The listing builds one solid part. Answer for the finished solid, in the listing's coordinates (mm). Give positions to 0.01 mm unless a question says otherwise; leave off trailing zeros. Loops run counter-clockwise (first coordinate to the right, second up) from the corner with the lowest first, then second, coordinate; pieces in that order, holes last. Notation, with made-up numbers: (9.25, 12) - (41.25, 12) arc R21 ccw to (41.25, 40) - close; hole circle Ø1 at (48, 9.5). An arc over 180 degrees is marked (long way). Write each question's results on one line, items separated by ' | '.
from build123d import *

# Parameters (mm, degrees)
SKETCH1_W           = 24
SKETCH1_H           = 30
BOSS_EXTRUDE1_DEPTH = 1.5
SKETCH2_R           = 1.55
CUT_EXTRUDE1_DEPTH  = 3
FILLET1_R           = 10
FILLET2_R           = 2


with BuildPart() as part:
    # Sketch1 → Boss-Extrude1 (new body, symmetric)
    with BuildSketch(Plane(origin=(0, 0, 0), x_dir=(1, 0, 0), z_dir=(0, 1, 0))):
        Polygon((-92, -95), (-92, -115), (12, -15), (-12, -15), (-12, 15), align=None)
        Rectangle(SKETCH1_W, SKETCH1_H)
    extrude(amount=BOSS_EXTRUDE1_DEPTH, both=True)

    # Sketch2 → Cut-Extrude1 (cut)
    with BuildSketch(Plane(origin=(0, 1.5, 0), x_dir=(1, 0, 0), z_dir=(0, 1, 0))):
        with Locations((6, 0)):
            Circle(SKETCH2_R)
        with Locations((-2, 0)):
            Circle(SKETCH2_R)
        with Locations((-47, -55)):
            Circle(SKETCH2_R)
    extrude(amount=-CUT_EXTRUDE1_DEPTH, mode=Mode.SUBTRACT)

    # Fillet1
    fillet1_edges = [part.edges().sort_by_distance(p)[0] for p in [
        (-92, 0, 95),
    ]]
    fillet(fillet1_edges, radius=FILLET1_R)

    # Fillet2
    fillet2_edges = [part.edges().sort_by_distance(p)[0] for p in [
        (-92, 0, 115),
    ]]
    fillet(fillet2_edges, radius=FILLET2_R)


solid = part.part
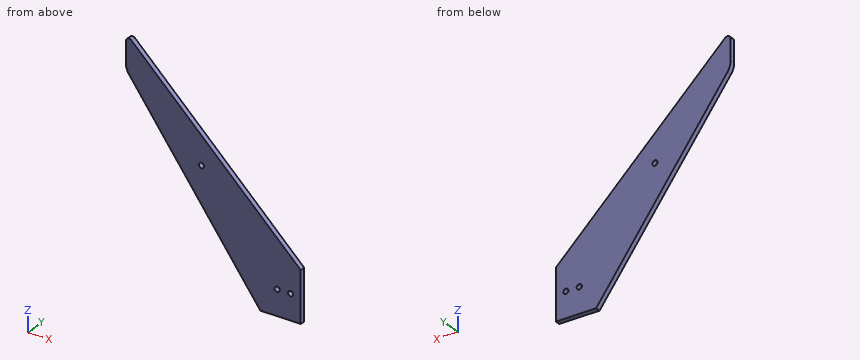
Item 1: A cutting plane is placed at C-C, the plane z = 0. Determine the outline of the cut face in (x, y), plus the area to 3 significant figures.
Values found:
outline: (-22.91, -1.5) - (-3.55, -1.5) - (-3.55, 1.5) - (-22.91, 1.5) - close; (-0.45, -1.5) - (4.45, -1.5) - (4.45, 1.5) - (-0.45, 1.5) - close; (7.55, -1.5) - (12, -1.5) - (12, 1.5) - (7.55, 1.5) - close | area: 86.1 mm²
Item 2: A cutting plane is placed at A-A, the plane y = 0.9. Determine the outline of the cut face in (x, z), plus the area to 3 significant figures.
Values found:
outline: (-92, 98.25) arc R10 ccw to (-90.09, 92.37) - (-12, -15) - (12, -15) - (12, 15) - (-88.61, 111.74) arc R2 ccw to (-92, 110.3) - close; hole circle Ø3.1 at (-47, 55); hole circle Ø3.1 at (-2, 0); hole circle Ø3.1 at (6, 0) | area: 3,890 mm²
Item 3: Find the intervals of material crossed by line 1 along X through (y, z) = (0.3, 0.5); line 2 along X through (y, z) = (-0.6, 0); line 3 along Z through (x, y) = (-2, 0.1), in increasing order. Write a range as [from, to].
Values found:
line 1: x = [-23.27, -3.47], [-0.53, 4.53], [7.47, 12] | line 2: x = [-22.91, -3.55], [-0.45, 4.45], [7.55, 12] | line 3: z = [-15, -1.55], [1.55, 28.46]
Item 4: A cutting plane is placed at B-B, the plane x = -2. Determine the outline of the cut face in (y, z).
Values found:
outline: (-1.5, -15) - (1.5, -15) - (1.5, -1.55) - (-1.5, -1.55) - close; (-1.5, 1.55) - (1.5, 1.55) - (1.5, 28.46) - (-1.5, 28.46) - close
Item 5: Flat-ended cylindrical pins translate along their axes: P1, Ø1.5, axis at x = -26.5, y = -0.5, coming from the +Z side; P2, Ø5, axis at x = 6, z = 0, coming from the -Y side; P3, Ø1.9, axis at x = -47, z = 55, coming from the +Y side. Find the tip coordinate at first contact, or state that the pin passes through.
Values found:
P1: stops at z = 52.74 | P2: stops at y = -1.5 | P3: passes through
Item 6: A cutting plane is placed at D-D, the plane x = -47. Determine the outline of the cut face in (y, z) (3 decimals).
Values found:
outline: (-1.5, 33.125) - (1.5, 33.125) - (1.5, 53.45) - (-1.5, 53.45) - close; (-1.5, 56.55) - (1.5, 56.55) - (1.5, 71.731) - (-1.5, 71.731) - close
